```python
from build123d import *

# Parameters (mm, degrees)
F0_W     = 95.25
F0_H     = 76.2
F0_W_2   = 88.9
F0_H_2   = 63.5
F1_DEPTH = 25.4
F2_W     = 88.9
F2_H     = 63.5
F3_DEPTH = 3.175


with BuildPart() as f1:
    # F0 (on Top) → F1 (new body)
    with BuildSketch(Plane.XY):
        with Locations((0, 3.175)):
            Rectangle(F0_W, F0_H)
        Rectangle(F0_W_2, F0_H_2, mode=Mode.SUBTRACT)
    extrude(amount=F1_DEPTH)

    # F2 (on Top) → F3 (join)
    with BuildSketch(Plane.XY):
        Rectangle(F2_W, F2_H)
    extrude(amount=F3_DEPTH)


solid = f1.part
```
The model under review builds one solid part; all positions refer to its coordinate system, in mm. A direction names the side the tool comes from. Round coordinates to 2 decimals unless told otherwise and drop trailing zeros. Loops run counter-clockwise (first coordinate to the right, second up) from the corner with the lowest first, then second, coordinate; pieces in that order, holes last. Notation, with made-up numbers: (66, 16.5) - (82, 16.5) arc R27 ccw to (82, 45.5) - close; hole circle Ø9 at (5.25, 32). An arc over 180 degrees is marked (long way). Write each question's results on one line, items separated by ' | '. Start each with the question number.
Q1. Wall thickness on line 1 along X through (y, z) = (9, 8.5) (3 decimals); line 2 along Y through (x, z) = (31.5, 6) (3 decimals); line 3 along Z through (x, y) = (19.5, -20) (3 decimals): over which ranges is each line inside the solid? List them lowest first. Write a range as [from, to].
Q2. Draft analysis for pull direction X (two halves, no side actions). For faces 3 (the flat face through (-1, 41.275, 13)), 4 (the flat face through (-47.625, 3, 13)), 5 (the flat face through (-1, 0, 3.175)), 6 (the flat face through (44.45, 0, 14)), state which applies: pulls with the +X half, pulls with the -X half, needs draft (parallel to the pull), parting line crosses it, or undercut.
Q3. Take a section at B-B on x = -38.5. Give the boundary of the cut face in (y, z) (3 decimals), plus the area to 3 significant figures.
Q4. Take a section at A-A on z = 8. Give the boundary of the cut face in (x, y) (3 decimals).
Q5. Tool access review of faces 1 (the flat face through (-1, 31.75, 14)), 2 (the flat face through (47.625, 3, 13)): name each direction out of +Z, -Z, +X, -X, +Y, -Y from which nothing blocks a thin tool from reaching the whole face with its end or side.
Q6. Take a section at C-C on y = -29. Give the boundary of the cut face in (x, z) (3 decimals), plus the area to 3 significant figures.
Q7. Insertion check: P1, Ø1.5, axis at x = 21, y = 28, coming from the -Z side; P2, Ø3, axis at x = -1.5, y = -16.5, coming from the +Z side (3 decimals). Each pin has a flat end and moves straight along its axis. Give the tip position at first contact, or say it passes through.
Data:
1) line 1: x = [-47.625, -44.45], [44.45, 47.625] | line 2: y = [-34.925, -31.75], [31.75, 41.275] | line 3: z = [0, 3.175]
2) face 3: needs draft | face 4: pulls with the -X half | face 5: undercut | face 6: undercut
3) outline: (-34.925, 0) - (41.275, 0) - (41.275, 25.4) - (31.75, 25.4) - (31.75, 3.175) - (-31.75, 3.175) - (-31.75, 25.4) - (-34.925, 25.4) - close | area: 524 mm²
4) outline: (-47.625, -34.925) - (47.625, -34.925) - (47.625, 41.275) - (-47.625, 41.275) - close; hole (-44.45, -31.75) - (44.45, -31.75) - (44.45, 31.75) - (-44.45, 31.75) - close
5) face 1: +Z | face 2: +Z, -Z, +X, +Y, -Y
6) outline: (-47.625, 0) - (47.625, 0) - (47.625, 25.4) - (44.45, 25.4) - (44.45, 3.175) - (-44.45, 3.175) - (-44.45, 25.4) - (-47.625, 25.4) - close | area: 444 mm²
7) P1: stops at z = 0 | P2: stops at z = 3.175
